```python
from build123d import *

# Parameters (mm, degrees)
F1_DEPTH = 1500


with BuildPart() as f1:
    # F0 (on Front) → F1 (new body)
    with BuildSketch(Plane.XZ):
        with BuildLine():
            Line((-52.329856, 0), (0, 0))
            Line((0, 0), (0, 2))
            Line((0, 2), (-52.329856, 2))
            ThreePointArc((-52.329856, 2), (-82.023376, 12.743672), (-97.967784, 40))
            Line((-97.967784, 40), (-100, 40))
            ThreePointArc((-100, 40), (-83.444333, 11.324743), (-52.329856, 0))
        make_face()
    extrude(amount=F1_DEPTH)

    # F2: F1 across plane


with BuildPart() as f1_1:
    add(f1.part)
    add(f1.part.mirror(Plane.YZ))


solid = f1_1.part
```
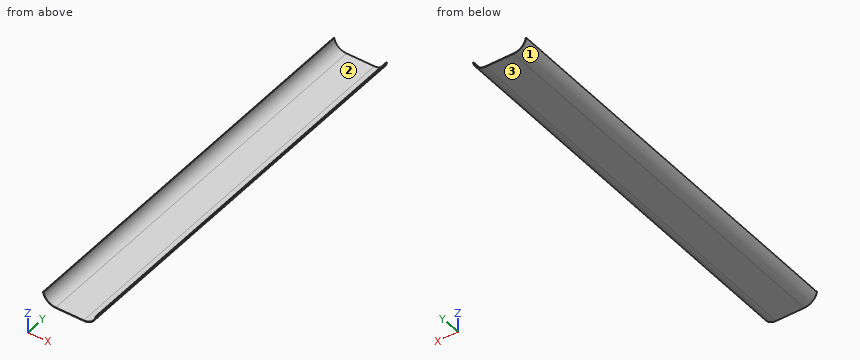
Work out the finished part from the listing and answer in its coordinate system (mm). Face numbers are marked on the shaded views. Give positions to 0.01 mm unless a question says otherwise; leave off trailing zeros. Loops run counter-clockwise (first coordinate to the right, second up) from the corner with the lowest first, then second, coordinate; pieces in that order, holes last. Notation, with made-up numbers: (-39.5, 53.25) -> (16.5, 53.25) arc R15 cw to (16.5, 82.25) -> close; hole circle Ø7 at (60.5, 29). An arc over 180 degrees is marked (long way). Put each result on its own line as item: value. Start each with the question number.
Item 1: The part is cut by section B-B (z = 13). Give the vertices of the cut face in (x, y), then the cut area to 3 significant figures.
Item 2: The part is cut by section A-A (y = -449). Give the vertices of the cut face in (x, z).
Item 3: The part is cut by section C-C (x = 21). Give the vertices of the cut face in (y, z).
Item 4: Find the intervals of material crossed by L1, parallel to Z at x = 5, y = -1191; L2, parallel to Z at x = 54.5, y = -940.5; L3, parallel to X at y = -595, z = 8, in increasing order. Write a range as [from, to].
Item 5: The part is cut by section D-D (x = -72). Give the vertices of the cut face in (y, z), then the cut area to 3 significant figures.
Item 6: The mould has two halves that part along X. Classify the marked faces 1, 2 and 3: released by +X, released by -X, zero draft, split by the parting line, or undercut.
Item 7: Each of these flat-tipped pins is pushed along its axis until it touches: P1, Ø8, axis at x = 75, y = -254, coming from the +Z side; P2, Ø4, axis at x = -16.5, y = -590, coming from the +Z side; P3, Ø1.5, axis at y = -1095.5, z = 24.5, coming from the +X side. Where does it stop, or does it pass through?
Answers below:
1. outline: (-85.34, -1500) -> (-82.33, -1500) -> (-82.33, 0) -> (-85.34, 0) -> close; (82.33, -1500) -> (85.34, -1500) -> (85.34, 0) -> (82.33, 0) -> close
1. area: 9,030 mm2
2. outline: (-100, 40) arc R48.41 ccw to (-52.33, 0) -> (52.33, 0) arc R48.41 ccw to (100, 40) -> (97.97, 40) arc R46.41 cw to (52.33, 2) -> (-52.33, 2) arc R46.41 cw to (-97.97, 40) -> close
3. outline: (-1500, 0) -> (0, 0) -> (0, 2) -> (-1500, 2) -> close
4. L1: [0, 2]
4. L2: [0.05, 2.05]
4. L3: [-78.98, -75.15], [75.15, 78.98]
5. outline: (-1500, 4.18) -> (0, 4.18) -> (0, 6.38) -> (-1500, 6.38) -> close
5. area: 3,300 mm2
6. face 1: released by -X
6. face 2: undercut
6. face 3: zero draft
7. P1: z = 10.43
7. P2: z = 2
7. P3: x = 94.84
